from build123d import *

# Parameters (mm, degrees)
BOSS_EXTRUDE1_DEPTH = 25
BOSS_EXTRUDE5_DEPTH = 15
SKETCH3_R           = 17.5
BOSS_EXTRUDE6_DEPTH = 15
SKETCH4_R           = 10
CUT_EXTRUDE1_DEPTH  = 20
SKETCH5_R           = 7.5
CUT_EXTRUDE2_DEPTH  = 80
CUT_EXTRUDE3_DEPTH  = 10
SKETCH7_R           = 17.5
BOSS_EXTRUDE7_DEPTH = 5
SKETCH8_R           = 7.5
CUT_EXTRUDE4_DEPTH  = 315


with BuildPart() as part:
    # Sketch1 → Boss-Extrude1 (new body)
    with BuildSketch(Plane.XY):
        Polygon((-60, 0), (-60, -5), (-50, -15), (-30, -15), (-30, -10), (-10, -10), (-10, -15), (10, -15), (20, -5), (20, 0), (0, 0), (0, 20), (20, 20), (20, 25), (10, 35), (-10, 35), (-10, 30), (-30, 30), (-30, 35), (-50, 35), (-60, 25), (-60, 20), (-40, 20), (-40, 0), align=None)
    extrude(amount=BOSS_EXTRUDE1_DEPTH)

    # Sketch2 → Boss-Extrude5 (add)
    with BuildSketch(Plane(origin=(0, 0, 0), x_dir=(-1, 0, 0), z_dir=(0, 0, -1))):
        Polygon((55, 20), (40, 20), (40, 0), (55, 0), (55, 5), (45, 5), (45, 15), (55, 15), align=None)
        Polygon((-15, 15), (-15, 20), (0, 20), (0, 0), (-15, 0), (-15, 5), (-5, 5), (-5, 15), align=None)
    extrude(amount=-BOSS_EXTRUDE5_DEPTH)

    # Sketch3 → Boss-Extrude6 (add)
    with BuildSketch(Plane.XY.offset(25)):
        with Locations((-20, 10)):
            Circle(SKETCH3_R)
    extrude(amount=BOSS_EXTRUDE6_DEPTH)

    # Sketch4 → Cut-Extrude1 (cut)
    with BuildSketch(Plane.XY.offset(40)):
        with Locations((-20, 10)):
            Circle(SKETCH4_R)
    extrude(amount=-CUT_EXTRUDE1_DEPTH, mode=Mode.SUBTRACT)

    # Sketch5 → Cut-Extrude2 (cut)
    with BuildSketch(Plane.XY.offset(20)):
        with Locations((-20, 10)):
            Circle(SKETCH5_R)
    extrude(amount=-CUT_EXTRUDE2_DEPTH, mode=Mode.SUBTRACT)

    # Sketch6 → Cut-Extrude3 (cut)
    with BuildSketch(Plane.XY.offset(40)):
        with BuildLine():
            Line((-36.160714286, 16.714261968), (-27.410714286, 16.714261968))
            ThreePointArc((-27.410714286, 16.714261968), (-30, 10), (-27.410714286, 3.285738032))
            Line((-27.410714286, 3.285738032), (-36.160714286, 3.285738032))
            ThreePointArc((-36.160714286, 3.285738032), (-37.5, 10), (-36.160714286, 16.714261968))
        make_face()
        with BuildLine():
            Line((-12.589285714, 16.714261968), (-3.839285714, 16.714261968))
            ThreePointArc((-3.839285714, 16.714261968), (-2.5, 10), (-3.839285714, 3.285738032))
            Line((-3.839285714, 3.285738032), (-12.589285714, 3.285738032))
            ThreePointArc((-12.589285714, 3.285738032), (-10, 10), (-12.589285714, 16.714261968))
        make_face()
    extrude(amount=-CUT_EXTRUDE3_DEPTH, mode=Mode.SUBTRACT)

    # Sketch7 → Boss-Extrude7 (add)
    with BuildSketch(Plane(origin=(0, 0, 0), x_dir=(-1, 0, 0), z_dir=(0, 0, -1))):
        with Locations(Location((20, 10, 0), (0, 0, 337.438671909))):
            Circle(SKETCH7_R)
    extrude(amount=BOSS_EXTRUDE7_DEPTH)

    # Sketch8 → Cut-Extrude4 (cut)
    with BuildSketch(Plane(origin=(0, 0, -5), x_dir=(-1, 0, 0), z_dir=(0, 0, -1))):
        with Locations(Location((20, 10, 0), (0, 0, 180))):
            Circle(SKETCH8_R)
    extrude(amount=-CUT_EXTRUDE4_DEPTH, mode=Mode.SUBTRACT)


solid = part.part
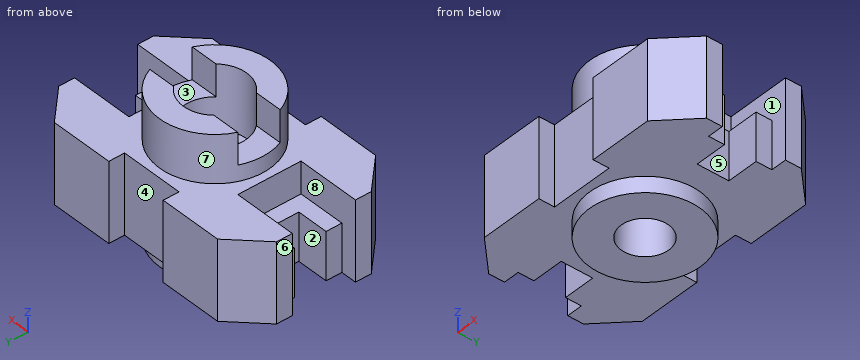
Geometry: final body of the model. Coordinates: model frame, mm. Face numbers are marked on the shaded views. A direction names the side the tool comes from. Give positions to 0.01 mm unless a question says otherwise; leave off trailing zeros. Loops run counter-clockwise (first coordinate to the right, second up) from the corner with the lowest first, then second, coordinate; pieces in that order, holes last. Notation, with made-up numbers: M 56.25,-22 L 80.25,-22 A22 cw 80.25,-3 Z; hole C 47.5,27 d11. An arc over 180 degrees is marked long. Put each result on its own line as item: value. Start each with the question number.
1) Cut plane B-B (y = 10). Output: boundary loops of the cut face in (x, z), then the cut area to 3 significant figures.
2) Access query for the marked faces 1, 2, 3, 4 and 5. Directions: +Z, -Z, +X, -X, +Y, -Y. A direction counts if a zero-diameter tool reaches every point of the face in a straight line with its end or side. Return the directions, or none.
3) Contact query for flat-ended pins moving along their axis: pin 1 (6 mm diameter, centred on x = -50.5, z = 10.5, fed in from -Y); pin 2 (4.5 mm diameter, centred on x = -7, z = 37.5, fed in from -Y); pin 3 (1 mm diameter, centred on y = -10, z = 13, fed in from +X); pin 4 (3 mm diameter, centred on y = 9, z = 6, fed in from -X). Output: stop coordinate, or through.
4) Pull-direction query (Y, two-part tool) for the marked faces 6, 7 and 8; classes: pulls with the +Y half, pulls with the -Y half, needs draft (parallel to the pull), parting line crosses it, or undercut.
5) Cut plane D-D (x = -20). Output: boundary loops of the cut face in (y, z).
6) Cut plane A-A (x = 11.5). Output: boundary loops of the cut face in (y, z), then the cut area to 3 significant figures.
7) Ray query, line 1 along Y through (x, z) = (-20, 10.25); line 2 along X through (y, z) = (10, 2.75); line 3 along Y through (x, z) = (-46.5, 23). Return the intervals inside material, ascending.
Verdict:
1. outline: M -45,0 L -37.5,0 L -37.5,-5 L -27.5,-5 L -27.5,20 L -30,20 L -30,30 L -37.5,30 L -37.5,25 L -40,25 L -40,15 L -45,15 Z; M -12.5,-5 L -2.5,-5 L -2.5,0 L 5,0 L 5,15 L 0,15 L 0,25 L -2.5,25 L -2.5,30 L -10,30 L -10,20 L -12.5,20 Z
1. area: 925 mm2
2. face 1: +Z, +X
2. face 2: +Z, -Z, -X
2. face 3: +Z, +X, -X
2. face 4: +Z, -Z, +Y
2. face 5: +Z, -Z, +X
3. pin 1: y = -15
3. pin 2: y = -3.81
3. pin 3: x = 15.5
3. pin 4: x = -45
4. face 6: needs draft
4. face 7: parting line crosses it
4. face 8: undercut
5. outline: M -10,0 L -7.5,0 L -7.5,-5 L 2.5,-5 L 2.5,20 L 0,20 L 0,40 L -7.5,40 L -7.5,25 L -10,25 Z; M 17.5,-5 L 27.5,-5 L 27.5,0 L 30,0 L 30,25 L 27.5,25 L 27.5,40 L 20,40 L 20,20 L 17.5,20 Z
6. outline: M -13.5,0 L 5,0 L 5,15 L 0,15 L 0,25 L -13.5,25 Z; M 15,0 L 33.5,0 L 33.5,25 L 20,25 L 20,15 L 15,15 Z
6. area: 825 mm2
7. line 1: -10 to 2.5, 17.5 to 30
7. line 2: -45 to -27.5, -12.5 to 5
7. line 3: -15 to 0, 20 to 35
